For this review, take the finished solid that the model builds, in its own axes (mm). A direction names the side the tool comes from. Round coordinates to 2 decimals unless told otherwise and drop trailing zeros. Order: outer loops, then holes, each group sorted by start corner. A loop starts at its lowest first (then second) coordinate and runs counter-clockwise, first axis right, second up. Notation, with made-up numbers: (17, -10) -> (40, -10) arc R16 ccw to (40, 1) -> close; hole circle Ø10 at (58, 14). An arc over 180 degrees is marked (long way). Answer in a Markdown table with one row per item.
Autodesk Inventor part; units mm, degrees
ref_plane "YZ Plane" through (0, 0, 0) normal (1, 0, 0) x (0, 1, 0)
ref_plane "XZ Plane" through (0, 0, 0) normal (0, 1, 0) x (-1, 0, 0)
ref_plane "XY Plane" through (0, 0, 0) normal (0, 0, 1) x (1, 0, 0)
sketch "Sketch1" plane through (0, 0, 0) normal (0, 0, 1) x (1, 0, 0)
  line L0 (-168, -100) -> (-210, -100)
  line L1 (-210, -100) -> (-210, 100)
  line L2 (-210, 100) -> (-168, 100)
  line L3 (-168, 100) -> (-168, -100)
  line L4 (-168, -100) -> (-210, 100) construction
  line L5 (-210, -100) -> (-168, 100) construction
  line L6 (-168, 0) -> (-168, 12.375)
  line L7 (-168, 12.375) -> (-174, 12.375)
  line L8 (-174, 12.375) -> (-174, -12.375)
  line L9 (-174, -12.375) -> (-168, -12.375)
  line L10 (-168, 12.375) -> (-168, 37.125)
  line L11 (-168, 37.125) -> (-174, 37.125)
  line L12 (-174, 37.125) -> (-174, 61.875)
  line L13 (-174, 61.875) -> (-168, 61.875)
  line L14 (-168, -12.375) -> (-168, -37.125)
  line L15 (-168, -37.125) -> (-174, -37.125)
  line L16 (-174, -37.125) -> (-174, -61.875)
  line L17 (-174, -61.875) -> (-168, -61.875)
  line L18 (-189, 0) -> (-189, 100)
  line L19 (-189, 0) -> (-173.1792, 0)
  line L20 (-210, 12.375) -> (-204, 12.375)
  line L21 (-204, 12.375) -> (-204, -12.375)
  line L22 (-204, -12.375) -> (-210, -12.375)
  line L23 (-210, 37.125) -> (-204, 37.125)
  line L24 (-204, 37.125) -> (-204, 61.875)
  line L25 (-204, 61.875) -> (-210, 61.875)
  line L26 (-210, -37.125) -> (-204, -37.125)
  line L27 (-204, -37.125) -> (-204, -61.875)
  line L28 (-204, -61.875) -> (-210, -61.875)
  line L29 (-185, -40) -> (-193, -40)
  line L30 (-193, -40) -> (-193, -100)
  line L31 (-193, -100) -> (-185, -100)
  line L32 (-185, -100) -> (-185, -40)
  line L33 (-185, -40) -> (-193, -100) construction
  line L34 (-193, -40) -> (-185, -100) construction
  point P0 (-210, 61.875)
  point P1 (-210, 37.125)
  point P2 (-210, 12.375)
  point P3 (-210, -12.375)
  point P4 (-210, -37.125)
  point P5 (-210, -61.875)
  point P6 (-189, -70)
  dimension "d18" = 42
  dimension "d19" = 200
  dimension "d20" = 12.375
  dimension "d21" = 6
  dimension "d22" = 24.75
  dimension "d23" = 24.75
  dimension "d24" = 6
  dimension "d25" = 24.75
  dimension "d26" = 24.75
  dimension "d27" = 6
  dimension "d28" = 24.75
  dimension "d31" = 8
  dimension "d32" = 60
  dimension "d34" = 0
  dimension "d35" = 21
extrude "Extrusion1" add sketch "Sketch1" along normal blind 6 contours L0 L32 L29 L30 L1 L28 L27 L26 L22 L21 L20 L23 L24 L25 L2 L18 L19 L8 L9 L3 L15 L16 L17 | L0 L30 L29 L32 | L7 L8 L19 L18 L2 L3 L13 L12 L11
extrude "Extrusion2" cut sketch "Sketch1" along normal blind 10 contours L0 L30 L29 L32
properties part number "Base_1"
Q1. Tool access review of faces 4 (the face through (-207, 12.375, 3)), 5 (the face through (-210, -81, 3)), 6 (the face through (-171, -61.875, 3)): name each direction out of +Z, -Z, +X, -X, +Y, -Y from which nothing blocks a thin tool from reaching the whole face with its end or side.
Answer key:
| item | result |
|---|---|
| face 4 | +Z, -Z, -X |
| face 5 | +Z, -Z, -X, +Y, -Y |
| face 6 | +Z, -Z, +X |
Q2. The part is to be moulded in two halves that separate along Y. For faces 1 (the face through (-171, -37.125, 3)), 2 (the face through (-189, -40, 3)), 3 (the face through (-185, -70, 3)), say which applies: +Y half, -Y half, draft (parallel to the pull), parting line (faces both ways), or undercut.
Answer key:
| item | result |
|---|---|
| face 1 | undercut |
| face 2 | -Y half |
| face 3 | draft |
Q3. To check wall thickness, follow probe 1 along Y at (x, z) = (-169.5, 3.35) (3 decimals); probe 2 along X at (y, z) = (-41, 2.2); probe 3 along X at (y, z) = (0.5, 3.15). State the ranges of each line that lie inside material, in increasing order.
Answer key:
| item | result |
|---|---|
| probe 1 | y = -100 to -61.875, -37.125 to -12.375, 12.375 to 37.125, 61.875 to 100 |
| probe 2 | x = -204 to -193, -185 to -174 |
| probe 3 | x = -204 to -174 |
Q4. Take a section at A-A, the plane y = -59.5. Write out the cut boundary in (x, z), then the cut area to 3 significant figures.
Answer key:
| item | result |
|---|---|
| outline | (-204, 0) -> (-193, 0) -> (-193, 6) -> (-204, 6) -> close; (-185, 0) -> (-174, 0) -> (-174, 6) -> (-185, 6) -> close |
| area | 132 mm^2 |
Q5. Clearance check with flat-ended pins moving along their axes: pin 1 Ø3 at (x, z) = (-188, 4) entering from -Y; pin 2 Ø10 at (x, y) = (-203, -33.5) entering from -Z; pin 3 Ø3 at (y, z) = (-5, 2.5) entering from -X. State where each tip first meets the part, or that it passes through.
Answer key:
| item | result |
|---|---|
| pin 1 | stops at y = -40 |
| pin 2 | stops at z = 0 |
| pin 3 | stops at x = -204 |
Q6. Take a section at B-B, the plane x = -207. Write out the cut boundary in (y, z) (3 decimals), then the cut area to 4 significant figures.
Answer key:
| item | result |
|---|---|
| outline | (-100, 0) -> (-61.875, 0) -> (-61.875, 6) -> (-100, 6) -> close; (-37.125, 0) -> (-12.375, 0) -> (-12.375, 6) -> (-37.125, 6) -> close; (12.375, 0) -> (37.125, 0) -> (37.125, 6) -> (12.375, 6) -> close; (61.875, 0) -> (100, 0) -> (100, 6) -> (61.875, 6) -> close |
| area | 754.5 mm^2 |
Q7. Take a section at D-D, the plane x = -189.5. Write out the cut boundary in (y, z).
Answer key:
| item | result |
|---|---|
| outline | (-40, 0) -> (100, 0) -> (100, 6) -> (-40, 6) -> close |
